Autodesk Inventor part; units mm, degrees
ref_plane "РабПлоскость1" through (25, 2, 0) normal (1, 0, 0) x (0, 0, -1)
ref_plane "РабПлоскость2" through (2, 12.5, 0) normal (0, -1, 0) x (1, 0, 0)
ref_plane "YZ Plane" through (0, 0, 0) normal (1, 0, 0) x (0, 1, 0)
sketch "Эскиз1" plane through (0, 0, 0) normal (0, 0, 1) x (1, 0, 0)
  line L0 (0, 0) -> (50, 0)
  line L1 (50, 0) -> (50, 25)
  line L2 (50, 25) -> (0, 25)
  line L3 (0, 25) -> (0, 0)
  dimension "d0" = 50
  dimension "d1" = 25
extrude "Выдавливание1" add sketch "Эскиз1" along normal blind 5.2
shell "Оболочка1" thickness 2 removed faces 1 at (16.6667, 16.6667, 0)
sketch "Эскиз2" plane through (0, 0, 5.2) normal (0, 0, 1) x (1, 0, 0)
  line L0 (50, 25) -> (0, 25)
  line L1 (25, 25) -> (25, 0)
  line L2 (0, 0) -> (50, 0)
  line L3 (25, 12.5) -> (12, 12.5)
  line L4 (0, 25) -> (0, 0)
  circle A0 centre (12, 12.5) radius 8.1
  circle A1 centre (38, 12.5) radius 8.1
  line L5 (25, 25) -> (25, 20)
  line L6 (21.75, 20) -> (28.25, 20) construction
  line L7 (21.75, 18) -> (28.25, 18)
  line L8 (28.25, 22) -> (21.75, 22)
  arc A2 (21.75, 22) -> (21.75, 18) centre (21.75, 20) ccw
  arc A3 (28.25, 18) -> (28.25, 22) centre (28.25, 20) ccw
  point P0 (25, 18)
  point P1 (25, 22)
  dimension "d5" = 13
  dimension "d6" = 16.2
  dimension "d9" = 5
  dimension "d10" = 3.25
  dimension "d11" = 4
extrude "Выдавливание2" cut sketch "Эскиз2" against normal through all contours L8 A3 L7 L1 | L1 L7 A2 L8 | A0 | A1
sketch "Эскиз5" plane through (48, 23, 3.2) normal (0, 0, -1) x (-1, 0, 0)
  line L0 (0, 0) -> (1.05, 0)
  line L1 (0, 0) -> (46, 0)
  line L2 (1.05, 0) -> (1.05, -1.05)
  circle A0 centre (1.05, -1.05) radius 1.05
  line L3 (2.1, -2.1) -> (0, -2.1)
  line L4 (0, -2.1) -> (0, 0)
  line L5 (0, 0) -> (2.1, 0)
  line L6 (2.1, 0) -> (2.1, -2.1)
  line L7 (2.1, -2.1) -> (0, 0) construction
  line L8 (0, -2.1) -> (2.1, 0) construction
  point P0 (48, -23)
  point P1 (1.05, -2.1)
  point P2 (2.1, -1.05)
  dimension "d17" = 1.05
  dimension "d18" = 1.05
extrude "Выдавливание4" add sketch "Эскиз5" along normal blind 1 contours L0 A0 L4 | L1 L6 A0 | A0 | A0 L3 L4
ref_plane "РабПлоскость1" through (25, 2, 0) normal (1, 0, 0) x (0, 0, -1)
ref_plane "РабПлоскость2" through (2, 12.5, 0) normal (0, -1, 0) x (1, 0, 0)
mirror "Зеркальное отражение1" about plane through (2, 12.5, 0) normal (0, -1, 0) of "Выдавливание4"
mirror "Зеркальное отражение2" about plane through (25, 2, 0) normal (1, 0, 0) of "Выдавливание4", "Зеркальное отражение1"
sketch "Эскиз19" plane through (0, 0, 0) normal (0, -1, 0) x (1, 0, 0)
  line L0 (0, 0) -> (50, 0)
  line L1 (50, 0) -> (50, 5.2)
  line L2 (0, 5.2) -> (50, 5.2)
  line L3 (0, 0) -> (0, 5.2)
extrude "Выдавливание14" add sketch "Эскиз19" along normal blind 5
sketch "Эскиз17" plane through (0, -5, 0) normal (0, -1, 0) x (1, 0, 0)
  line L0 (40.15, 5.2) -> (9.85, 5.2)
  line L1 (9.85, 5.2) -> (9.85, -27.35)
  line L2 (9.85, -27.35) -> (40.15, -27.35)
  line L3 (40.15, -27.35) -> (40.15, 5.2)
  line L4 (50, 5.2) -> (0, 5.2)
  point P0 (0, 0)
  point P1 (25, 5.2)
  dimension "d77" = 30.3
  dimension "d78" = 32.55
extrude "Выдавливание13" add sketch "Эскиз17" against normal blind 3
sketch "Эскиз18" plane through (45.9, 2, 2.2) normal (0, 1, 0) x (1, 0, 0)
  line L0 (-10.3, 25.55) -> (-31.5, 25.55)
  line L1 (-20.9, 25.55) -> (-20.9, 29.55)
  line L2 (-36.05, 29.55) -> (-5.75, 29.55)
  point P0 (-45.9, 2.2)
  dimension "d81" = 4
  dimension "d82" = 21.2
hole "Отверстие4" at (35.6, 2, -23.35) at (14.4, 2, -23.35) direction (0, -1, 0) diameter 3.2 end through all
fillet "Сопряжение4" radius 5.05 2 edges at (40.15, -3.5, -27.35) (9.85, -3.5, -27.35)
fillet "Сопряжение5" radius 9.85 2 edges at (40.15, -3.5, 0) (9.85, -3.5, 0)
chamfer "Фаска1" distance 4 angle 45 2 edges at (45.075, -2, 0) (4.9251, -2, 0)
properties part number "Крепление ультрасоника заднее"
For this review, take the finished solid that the model builds, in its own axes (mm). A direction names the side the tool comes from. Coordinates: 2 decimals unless noted, no trailing zeros. Loops run counter-clockwise (first coordinate to the right, second up) from the corner with the lowest first, then second, coordinate; pieces in that order, holes last.
1. For line 1 (Y direction, x = 26.5, z = 3); line 2 (X direction, y = -3.6, z = -23.35); line 3 (Y direction, x = 38, z = 4.4), list the stretches that pass through material, from the lowest coordinate up.
2. For faces 4 (the cylindrical face through (30.25, 19.96, 4.21)), 5 (the cylindrical face through (5.738, -2.327, -1.844)), 6 (the flat face through (25, 13, 3.2)), list the 3-axis set-ups (+Z, -Z, +X, -X, +Y, -Y) from which the entire face can be reached by the end or side of a thin tool; tool diameter is ignored.
3. Mouldability with a two-part tool opening along X and no side actions: class faces 1 (the flat face through (25, -2, -16)), 2 (the cylindrical face through (37.02, -3.52, -22.61)), 3 (the flat face through (40.15, -4, -16)) as +X half, -X half, draft (parallel to the pull), parting line (faces both ways), or undercut.
4. Add section A-A, the plane y = 12.5. Give the boundary of the cut face in (x, z).
5. Insertion check: P1, Ø5, axis at x = 14, y = 5.5, coming from the -Z side; P2, Ø1.7, axis at x = 3.5, y = 3.5, coming from the -Z side; P3, Ø5, axis at x = 39, z = -8, coming from the +Y side; P4, Ø14.5, axis at x = 38, y = 12.5, coming from the +Z side. Each pin has a flat end and moves straight along its axis. Give the tip position at first contact, or say it passes through.
6. Add section D-D, the plane y = 20. Give the boundary of the cut face in (x, z), then the cut area to 3 significant figures.
7. Add section C-C, the plane z = -23.35. Give the boundary of the cut face in (x, y).
Result:
1. line 1: y = -5 to 2, 23 to 25
1. line 2: x = 9.96 to 12.8, 16 to 34, 37.2 to 40.04
1. line 3: y = -5 to 4.4, 20.6 to 25
2. face 4: +Z, -Z
2. face 5: -Z, -X, +Y, -Y
2. face 6: -Z
3. face 1: draft
3. face 2: undercut
3. face 3: +X half
4. outline: (0, 0) - (2, 0) - (2, 3.2) - (3.9, 3.2) - (3.9, 5.2) - (0, 5.2) - close; (20.1, 3.2) - (29.9, 3.2) - (29.9, 5.2) - (20.1, 5.2) - close; (46.1, 3.2) - (48, 3.2) - (48, 0) - (50, 0) - (50, 5.2) - (46.1, 5.2) - close
5. P1: stops at z = 3.2
5. P2: stops at z = 2.2
5. P3: stops at y = -2
5. P4: passes through
6. outline: (0, 0) - (2, 0) - (2, 3.2) - (8.94, 3.2) - (8.94, 5.2) - (0, 5.2) - close; (15.06, 3.2) - (19.75, 3.2) - (19.75, 5.2) - (15.06, 5.2) - close; (30.25, 3.2) - (34.94, 3.2) - (34.94, 5.2) - (30.25, 5.2) - close; (41.06, 3.2) - (48, 3.2) - (48, 0) - (50, 0) - (50, 5.2) - (41.06, 5.2) - close
6. area: 67.3 mm2
7. outline: (9.96, -5) - (12.8, -5) - (12.8, -2) - (9.96, -2) - close; (16, -5) - (34, -5) - (34, -2) - (16, -2) - close; (37.2, -5) - (40.04, -5) - (40.04, -2) - (37.2, -2) - close
